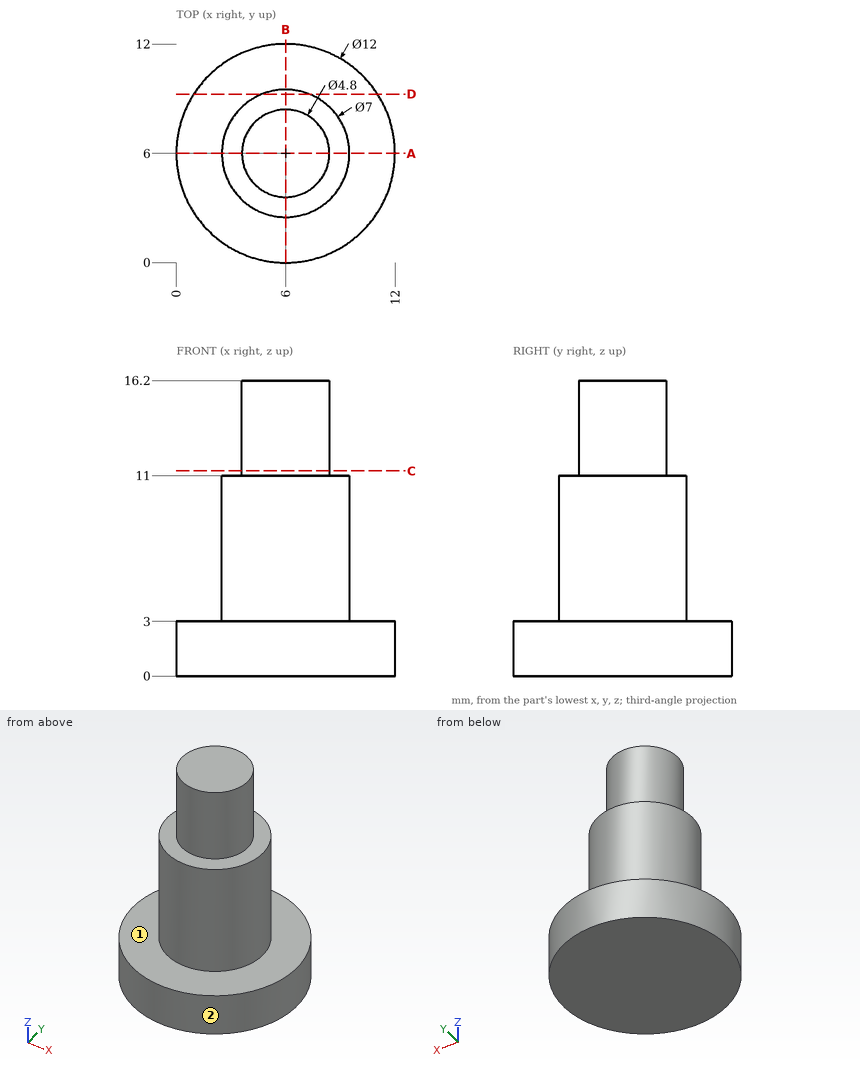
Here's the drawing with two shaded views (mm, measured from the low corner). I have some questions. A direction names the side the tool comes from. Give positions to 0.01 mm unless a question says otherwise; leave off trailing zeros. Write each loop counter-clockwise with the first axis right and the second up, starting at its lowest first coordinate (ties: lowest second). Pieces come first, ordered by that corner, then holes. Notation, with made-up numbers: (23.5, 5) -> (75.5, 5) arc R24 cw to (75.5, 26) -> close; hole circle Ø2 at (65, 85). An arc over 180 degrees is marked (long way). Use one line per item in the form item = value.
1) Suppose I cut it at A-A (y = 6). Please give me the cut outline in (x, z), and give its area (3 significant figures).
Verdict:
outline = (0, 0) -> (12, 0) -> (12, 3) -> (9.5, 3) -> (9.5, 11) -> (8.4, 11) -> (8.4, 16.2) -> (3.6, 16.2) -> (3.6, 11) -> (2.5, 11) -> (2.5, 3) -> (0, 3) -> close
area = 117 mm2
2) I'm going to push flat-ended pins straight in: pin 1 (3 mm diameter, centred on y = 1.5, z = 3, fed in from -X); pin 2 (2 mm diameter, centred on x = 7.5, z = 2.5, fed in from +Y); pin 3 (6 mm diameter, centred on y = 2.5, z = 3.5, fed in from +X). Where does each tip first touch, or does it pass through?
Verdict:
pin_1 = 0.8
pin_2 = 11.98
pin_3 = 11.98
3) On a 3-axis mill with a long thin cutter (end or side, diameter ignored), from which of +Z, -Z, +X, -X, +Y, -Y can I reach the whole of each face in a straight line? I mean the marked faces 1 and 2. Say none if no direction works.
Verdict:
face_1 = +Z
face_2 = +Z, -Z
4) Suppose I cut it at D-D (y = 9.25). Please give me the cut outline in (x, z).
Verdict:
outline = (0.96, 0) -> (11.04, 0) -> (11.04, 3) -> (7.3, 3) -> (7.3, 11) -> (4.7, 11) -> (4.7, 3) -> (0.96, 3) -> close
5) Suppose I cut it at C-C (z = 11.25). Please give me the cut outline in (x, y).
Verdict:
outline = circle Ø4.8 at (6, 6)
6) If I drill on L1, parallel to Z at x = 7, y = 2; L2, parallel to Z at x = 3.5, y = 4.5; L3, parallel to Y at x = 4.25, z = 10, over which ranges is the centre line in solid material (lowest first)? Write a range as [from, to].
Verdict:
L1 = [0, 3]
L2 = [0, 11]
L3 = [2.97, 9.03]
